```python
from build123d import *

# Parameters (mm, degrees)
SKETCH_2_R          = 27
EXTRUDE_1_DEPTH     = 18
SKETCH_5_R          = 14.1
CUT_EXTRUDE_1_DEPTH = 5
CUT_EXTRUDE_START   = 6
SKETCH_6_R          = 43.385104725
SKETCH_6_R_2        = 20
CUT_EXTRUDE_2_DEPTH = 37.213741838
CUT_EXTRUDE_START_2 = 8
SKETCH_7_R          = 38.171237221
SKETCH_7_R_2        = 17.5
CUT_EXTRUDE_3_DEPTH = 35.213741838
SKETCH_8_R          = 1.75
CUT_EXTRUDE_4_DEPTH = 43.213741838
CUT_EXTRUDE_START_3 = 3
SKETCH_9_R          = 3.25
CUT_EXTRUDE_5_DEPTH = 40.213741838
CHAMFER1_SIZE       = 1
CHAMFER2_SIZE       = 1
CHAMFER3_SIZE       = 1
CHAMFER4_SIZE       = 1
SKETCH_10_R         = 2.5
CUT_EXTRUDE_6_DEPTH = 2.5
SKETCH_11_R         = 8
SKETCH_11_R_2       = 4
CUT_EXTRUDE_7_DEPTH = 4


with BuildPart() as part:
    # Эскиз2 → Бобышка-Вытянуть1 (new body)
    with BuildSketch(Plane(origin=(0, 0, 0), x_dir=(1, 0, 0), z_dir=(0, 1, 0))):
        with Locations(Location((0, 0, 0), (0, 0, 270))):
            Circle(SKETCH_2_R)
    extrude(amount=EXTRUDE_1_DEPTH)

    # Эскиз5 → Вырез-Вытянуть1 (cut)
    with BuildSketch(Plane(origin=(0, 0, 0), x_dir=(1, 0, 0), z_dir=(0, 1, 0))):
        with Locations(Location((0, 0, 0), (0, 0, 270))):
            Circle(SKETCH_5_R)
    extrude(amount=CUT_EXTRUDE_1_DEPTH, mode=Mode.SUBTRACT)

    # Эскиз6 → Вырез-Вытянуть2 (cut, through all)
    with BuildSketch(Plane(origin=(0, 0, 0), x_dir=(1, 0, 0), z_dir=(0, 1, 0)).offset(CUT_EXTRUDE_START)):
        Circle(SKETCH_6_R)
        with Locations(Location((0, 0, 0), (0, 0, 270))):
            Circle(SKETCH_6_R_2, mode=Mode.SUBTRACT)
    extrude(amount=CUT_EXTRUDE_2_DEPTH, mode=Mode.SUBTRACT)

    # Эскиз7 → Вырез-Вытянуть3 (cut, through all)
    with BuildSketch(Plane(origin=(0, 0, 0), x_dir=(1, 0, 0), z_dir=(0, 1, 0)).offset(CUT_EXTRUDE_START_2)):
        Circle(SKETCH_7_R)
        with Locations(Location((0, 0, 0), (0, 0, 270))):
            Circle(SKETCH_7_R_2, mode=Mode.SUBTRACT)
    extrude(amount=CUT_EXTRUDE_3_DEPTH, mode=Mode.SUBTRACT)

    # Эскиз8 → Вырез-Вытянуть4 (cut, through all)
    with BuildSketch(Plane(origin=(0, 0, 0), x_dir=(1, 0, 0), z_dir=(0, 1, 0))):
        with Locations(Location((0, 22, 0), (0, 0, 270))):
            Circle(SKETCH_8_R)
        with Locations(Location((22, 0, 0), (0, 0, 270))):
            Circle(SKETCH_8_R)
        with Locations(Location((0, -22, 0), (0, 0, 270))):
            Circle(SKETCH_8_R)
        with Locations(Location((-22, 0, 0), (0, 0, 270))):
            Circle(SKETCH_8_R)
    extrude(amount=CUT_EXTRUDE_4_DEPTH, mode=Mode.SUBTRACT)

    # Эскиз9 → Вырез-Вытянуть5 (cut, through all)
    with BuildSketch(Plane(origin=(0, 0, 0), x_dir=(1, 0, 0), z_dir=(0, 1, 0)).offset(CUT_EXTRUDE_START_3)):
        with Locations(Location((0, 22, 0), (0, 0, 318.602722353))):
            Circle(SKETCH_9_R)
        with Locations(Location((22, 0, 0), (0, 0, 131.397277647))):
            Circle(SKETCH_9_R)
        with Locations(Location((0, -22, 0), (0, 0, 138.602722353))):
            Circle(SKETCH_9_R)
        with Locations(Location((-22, 0, 0), (0, 0, 48.602722353))):
            Circle(SKETCH_9_R)
    extrude(amount=CUT_EXTRUDE_5_DEPTH, mode=Mode.SUBTRACT)

    # Chamfer1
    chamfer1_edges = [part.edges().sort_by_distance(p)[0] for p in [
        (0, 0, -14.1),
    ]]
    chamfer(chamfer1_edges, length=CHAMFER1_SIZE)

    # Chamfer2
    chamfer2_edges = [part.edges().sort_by_distance(p)[0] for p in [
        (0, 18, -17.5),
    ]]
    chamfer(chamfer2_edges, length=CHAMFER2_SIZE)

    # Chamfer3
    chamfer3_edges = [part.edges().sort_by_distance(p)[0] for p in [
        (0, 0, -27),
    ]]
    chamfer(chamfer3_edges, length=CHAMFER3_SIZE)

    # Chamfer4
    chamfer4_edges = [part.edges().sort_by_distance(p)[0] for p in [
        (0, 6, -27),
    ]]
    chamfer(chamfer4_edges, length=CHAMFER4_SIZE)

    # Эскиз10 → Вырез-Вытянуть6 (cut)
    with BuildSketch(Plane(origin=(0, 18, 0), x_dir=(1, 0, 0), z_dir=(0, 1, 0))):
        with Locations(Location((0, 0, 0), (0, 0, 270))):
            Circle(SKETCH_10_R)
    extrude(amount=-CUT_EXTRUDE_6_DEPTH, mode=Mode.SUBTRACT)

    # Эскиз11 → Вырез-Вытянуть7 (cut)
    with BuildSketch(Plane(origin=(0, 18, 0), x_dir=(1, 0, 0), z_dir=(0, 1, 0))):
        with Locations(Location((0, 0, 0), (0, 0, 270))):
            Circle(SKETCH_11_R)
        with Locations(Location((0, 0, 0), (0, 0, 270))):
            Circle(SKETCH_11_R_2, mode=Mode.SUBTRACT)
    extrude(amount=-CUT_EXTRUDE_7_DEPTH, mode=Mode.SUBTRACT)


solid = part.part
```
Work out the finished part from the listing and answer in its coordinate system (mm). A direction names the side the tool comes from. Give positions to 0.01 mm unless a question says otherwise; leave off trailing zeros. One line per question, with ' | ' between items.
(1) A tool of negligible diameter and unlimited length cuts with its end or side. For faces 1 (the face through (0.782, 4.909, 18.845)), 2 (the face through (14.273, 6.986, -14.01)), 3 (the face through (-14.01, 6.986, -14.273)), from which of +Z, -Z, +X, -X, +Y, -Y can it reach the whole face along a straight path? Write none if from no direction.
Recorded:
face 1: +Y | face 2: -Z, +X, +Y | face 3: -Z, -X, +Y
(2) The part is cut by section A-A (x = 0). Count the separate pieces of the cut face and the enclosed holes in it, then the cut area to 4 significant figures.
Recorded:
separate pieces: 3 | enclosed holes: 0 | area: 499.5 mm²
(3) Straight lines are drawn through the part: probe 1 along X at (y, z) = (16.35, 0); probe 2 along X at (y, z) = (17.1, 0); probe 3 along Y at (x, z) = (-3, -8.5). For each, find the intervals that lie inside material, in ascending order.
Recorded:
probe 1: x = -17.5 to -8, -4 to -2.5, 2.5 to 4, 8 to 17.5 | probe 2: x = -17.4 to -8, -4 to -2.5, 2.5 to 4, 8 to 17.4 | probe 3: y = 5 to 18
(4) The mould has two halves that part along X. Classify faces 4 (the face through (19.22, 4.91, -1.68)), 5 (the face through (-26.36, 2.97, -5.85)), 6 (the face through (2, 18, 2)): +X half, -X half, draft (parallel to the pull), parting line (faces both ways), or undercut.
Recorded:
face 4: undercut | face 5: parting line | face 6: draft
(5) Each of these flat-tipped pins is pushed along its axis until it touches: pin 1 Ø1.5 at (x, z) = (18, 16) entering from +Y; pin 2 Ø10 at (x, y) = (-20.5, 14) entering from +Z; pin 3 Ø4 at (y, z) = (15.5, -3.5) entering from +X. Where does it stop, or does it pass through?
Recorded:
pin 1: stops at y = 6 | pin 2: stops at z = 8.12 | pin 3: stops at x = 17.44
